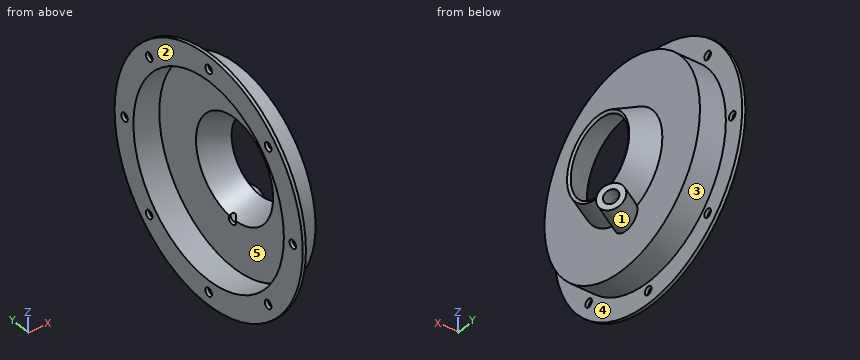
from build123d import *

# Parameters (mm, degrees)
SKETCH2_R                       = 3.302
CUT_EXTRUDE1_DEPTH              = 2.54
BOSS_EXTRUDE1_REACH             = 85.185
SKETCH3_R                       = 10.16
SKETCH3_R_2                     = 5.55625
BOSS_EXTRUDE1_DIRECTION_2_DEPTH = 10.16
CUT_EXTRUDE2_REACH              = 85.185
SKETCH3_7_R                     = 3.175


with BuildPart() as part:
    # Sketch1 → Revolve1 (revolve)
    with BuildSketch(Plane.XY):
        Polygon((0, 95.25), (2.54, 95.25), (2.54, 78.74), (22.86, 78.74), (22.86, 40.64), (41.745574265, 31.509467488), (40.64, 29.2227), (20.32, 39.046728544), (20.32, 76.2), (0, 76.2), align=None)
    revolve(axis=Axis((0, 0, 0), (1, 0, 0)))

    # Sketch2 → Cut-Extrude1 (cut)
    with BuildSketch(Plane(origin=(2.54, 0, 0), x_dir=(0, 0, -1), z_dir=(1, 0, 0))):
        with Locations((0, 85.217)):
            Circle(SKETCH2_R)
        with Locations((60.257518572, 60.257518572)):
            Circle(SKETCH2_R)
        with Locations((85.217, 0)):
            Circle(SKETCH2_R)
        with Locations((60.257518572, -60.257518572)):
            Circle(SKETCH2_R)
        with Locations((0, -85.217)):
            Circle(SKETCH2_R)
        with Locations((-60.257518572, -60.257518572)):
            Circle(SKETCH2_R)
        with Locations((-85.217, 0)):
            Circle(SKETCH2_R)
        with Locations((-60.257518572, 60.257518572)):
            Circle(SKETCH2_R)
    extrude(amount=-CUT_EXTRUDE1_DEPTH, mode=Mode.SUBTRACT)

    # Sketch3 → Boss-Extrude1 (add, up to next)
    with BuildSketch(Plane(origin=(30.795863359, 17.78, 0), x_dir=(0, 0, 1), z_dir=(0.866025404, 0.5, 0)), mode=Mode.PRIVATE) as boss_extrude1_sk1:
        with Locations((-40.474297606, 8.255)):
            Circle(SKETCH3_R)
        with Locations((-40.474297606, 8.255)):
            Circle(SKETCH3_R_2, mode=Mode.SUBTRACT)
    boss_extrude1_tool1 = extrude(boss_extrude1_sk1.sketch, amount=-BOSS_EXTRUDE1_REACH, mode=Mode.PRIVATE) - part.part
    add(boss_extrude1_tool1.solids().sort_by_distance((34.923363, 10.63096, -50.346929))[0])

    # Sketch3 → Boss-Extrude1 direction 2 (add)
    with BuildSketch(Plane(origin=(30.795863359, 17.78, 0), x_dir=(0, 0, 1), z_dir=(0.866025404, 0.5, 0))):
        with Locations((-40.474297606, 8.255)):
            Circle(SKETCH3_R)
        with Locations((-40.474297606, 8.255)):
            Circle(SKETCH3_R_2, mode=Mode.SUBTRACT)
    extrude(amount=BOSS_EXTRUDE1_DIRECTION_2_DEPTH)

    # Sketch3_7 → Cut-Extrude2 (cut, up to next)
    with BuildSketch(Plane(origin=(30.795863359, 17.78, 0), x_dir=(0, 0, 1), z_dir=(0.866025404, 0.5, 0)), mode=Mode.PRIVATE) as cut_extrude2_sk1:
        with Locations((-40.474297606, 8.255)):
            Circle(SKETCH3_7_R)
    cut_extrude2_tool1 = extrude(cut_extrude2_sk1.sketch, amount=-CUT_EXTRUDE2_REACH, mode=Mode.PRIVATE) & part.part
    add(cut_extrude2_tool1.solids().sort_by_distance((34.923363, 10.63096, -40.474298))[0], mode=Mode.SUBTRACT)


solid = part.part
Verification items for the finished model (mm, model axes). Face numbers are marked on the shaded views. A direction names the side the tool comes from. Give positions to 0.01 mm unless a question says otherwise; leave off trailing zeros. Write each loop counter-clockwise with the first axis right and the second up, starting at its lowest first coordinate (ties: lowest second). Pieces come first, ordered by that corner, then holes.
(1) Mould release check, pull along Z, two halves, no side actions. Record for the marked faces 1, 2 and 3: +Z half, -Z half, draft (parallel to the pull), parting line (faces both ways), or undercut.
(2) Cross-section at B-B (x = 8.5). Enter the section's corners in (y, z), plus the area to 3 significant figures.
(3) Access from +Z, -Z, +X, -X, +Y, -Y to the whole of each face (thin tool, end or side, straight path). Record for the marked faces 4 and 5.
(4) Gauge pin test, flat ends, axial feed: pin 1 (8.5 mm diameter, centred on y = 0, z = 85.217, fed in from +X); pin 2 (5 mm diameter, centred on x = 34, z = -4, fed in from +Y); pin 3 (1 mm diameter, centred on y = 36, z = -42.5, fed in from +X). Record the tip position at first contact, or that the pin passes through.
(5) Cross-section at C-C (y = -47). Enter the section's corners in (x, z), plus the area to 3 significant figures.
(6) Material ranges on line 1 (Z direction, x = 10.5, y = 0); line 2 (X direction, y = -34, z = 50.5); line 3 (Y direction, x = 19.5, z = -58), recorded low to high.
(7) Cross-section at D-D (z = 51). Enter the section's corners in (x, y).
(8) Cross-section at A-A (z = 0). Enter the section's corners in (x, y) (3 decimals).
Worked out:
1. face 1: undercut
1. face 2: draft
1. face 3: parting line
2. outline: circle Ø157.48 at (0, 0); hole circle Ø152.4 at (0, 0)
2. area: 1,240 mm2
3. face 4: +X
3. face 5: -X
4. pin 1: stops at x = 2.54
4. pin 2: stops at y = 36.27
4. pin 3: stops at x = 22.86
5. outline: (0, -82.85) - (2.54, -82.85) - (2.54, -63.17) - (22.86, -63.17) - (22.86, 63.17) - (2.54, 63.17) - (2.54, 82.85) - (0, 82.85) - (0, 59.98) - (20.32, 59.98) - (20.32, -59.98) - (0, -59.98) - close
5. area: 551 mm2
6. line 1: z = -78.74 to -76.2, 76.2 to 78.74
6. line 2: x = 20.32 to 22.86
6. line 3: y = -53.25 to -49.42, 49.42 to 53.25
7. outline: (0, -80.45) - (2.54, -80.45) - (2.54, -59.99) - (22.86, -59.99) - (22.86, 59.99) - (2.54, 59.99) - (2.54, 80.45) - (0, 80.45) - (0, 56.62) - (20.32, 56.62) - (20.32, -56.62) - (0, -56.62) - close
8. outline: (0, -95.25) - (2.54, -95.25) - (2.54, -88.519) - (0, -88.519) - close; (0, -81.915) - (2.54, -81.915) - (2.54, -78.74) - (22.86, -78.74) - (22.86, -40.64) - (41.746, -31.509) - (40.64, -29.223) - (20.32, -39.047) - (20.32, -76.2) - (0, -76.2) - close; (0, 76.2) - (20.32, 76.2) - (20.32, 39.047) - (40.64, 29.223) - (41.746, 31.509) - (22.86, 40.64) - (22.86, 78.74) - (2.54, 78.74) - (2.54, 81.915) - (0, 81.915) - close; (0, 88.519) - (2.54, 88.519) - (2.54, 95.25) - (0, 95.25) - close
